Here's how the part is built. I have some questions about the finished solid (model axes, mm). A direction names the side the tool comes from. Coordinates: 2 decimals unless noted, no trailing zeros. Loops run counter-clockwise (first coordinate to the right, second up) from the corner with the lowest first, then second, coordinate; pieces in that order, holes last. Notation, with made-up numbers: (54, 18) - (68, 18) arc R33 ccw to (68, 56) - close; hole circle Ø3 at (48.25, 87.5). An arc over 180 degrees is marked (long way). Use a Markdown table: item, result.
```python
from build123d import *

# Parameters (mm, degrees)
BOX_W                     = 0.6
BOX_H                     = 0.4
BOX_DEPTH                 = 2.5
BOX001_W                  = 0.6
BOX001_H                  = 0.4
BOX001_DEPTH              = 2.5
CYLINDER011_R             = 5.5
CYLINDER011_DEPTH         = 2
BOX002_W                  = 6
BOX002_H                  = 15
BOX002_DEPTH              = 0.5
FILLET006_R               = 0.3
FUSION004_PLACEMENT_ANGLE = 90


with BuildPart() as cubo001:
    # Box → Box (new body)
    with BuildSketch(Plane(origin=(2.95, -0.2, -2), x_dir=(1, 0, 0), z_dir=(0, 0, 1))):
        with Locations((0.3, 0.2)):
            Rectangle(BOX_W, BOX_H)
    extrude(amount=BOX_DEPTH)


with BuildPart() as cubo002:
    # Box001 → Box001 (new body)
    with BuildSketch(Plane(origin=(-3.55, -0.2, -2), x_dir=(1, 0, 0), z_dir=(0, 0, 1))):
        with Locations((0.3, 0.2)):
            Rectangle(BOX001_W, BOX001_H)
    extrude(amount=BOX001_DEPTH)


with BuildPart() as interior:
    # Cylinder011 → Cylinder011 (new body)
    with BuildSketch(Plane.XY):
        Circle(CYLINDER011_R)
    extrude(amount=CYLINDER011_DEPTH)

    # Fusion: union Cubo001, Cubo002
    add(cubo001.part)
    add(cubo002.part)


with BuildPart() as interior_1:
    # Fusion placement: moved
    add(interior.part.moved(Location((0, 0, 0.5))))


with BuildPart() as cubo:
    # Box002 → Box002 (new body)
    with BuildSketch(Plane(origin=(-3, -7, 0), x_dir=(1, 0, 0), z_dir=(0, 0, 1))):
        with Locations((3, 7.5)):
            Rectangle(BOX002_W, BOX002_H)
    extrude(amount=BOX002_DEPTH)


with BuildPart() as obj1:
    # Sketch004 → Revolution001 (revolve)
    with BuildSketch(Plane.XZ):
        Polygon((5.5, 2.5), (5.5, 0), (6, 0), (6, 2), (5.75, 2), (5.75, 2.5), align=None)
    revolve(axis=Axis((0, 0, 0), (0, 0, 1)))

    # Cut013: cut Cubo
    add(cubo.part, mode=Mode.SUBTRACT)


with BuildPart() as buzzersensor:
    # Sketch003 → Revolution (revolve)
    with BuildSketch(Plane.XZ):
        Polygon((1.3, 9.57124), (6, 9.57124), (6, 2.17124), (5.75, 2.17124), (5.75, 2.57124), (5.5, 2.57124), (5.5, 9.07124), (1.3, 9.07124), align=None)
    revolve(axis=Axis((0, 0, 0), (0, 0, 1)))

    # Fillet006
    fillet006_edges = [buzzersensor.edges().sort_by_distance(p)[0] for p in [
        (-6, 0, 9.57124),
    ]]
    fillet(fillet006_edges, radius=FILLET006_R)

    # Fusion004: union Interior, obj1
    add(interior_1.part)
    add(obj1.part)


with BuildPart() as buzzersensor_1:
    # Fusion004 placement: moved
    add(buzzersensor.part.moved(Location((6, 2.7, 1))).rotate(Axis((6, 2.7, 1), (0, 0, 1)), FUSION004_PLACEMENT_ANGLE))


solid = buzzersensor_1.part
```
Q1. Please list where these lines run through material, in increasing order: L1, parallel to Z at x = 3.25, y = 5.75; L2, parallel to X at y = 2.7, z = 10.25; L3, parallel to X at y = 2.7, z = 8.5. Write a range as from..to.
Check values:
| item | result |
|---|---|
| L1 | 1.5..3.5, 10.07..10.57 |
| L2 | 0..4.7, 7.3..12 |
| L3 | 0..0.5, 11.5..12 |
Q2. Which directions (+Z, -Z, +X, -X, +Y, -Y) give clear straight access to the entire face, cutting with the end or side of a thin tool? Please do faces 1 (the face through (6, 1, 10.071)), 2 (the face through (6.1, 8.2, 1.2)), 3 (the face through (7.27, 2.42, 10.32)), 4 (the face through (11.323, 5.469, 6.672)).
Check values:
| item | result |
|---|---|
| face 1 | none |
| face 2 | -Z |
| face 3 | +Z |
| face 4 | +Z, -Z |
Q3. Will these pins go through, and if not, where does the flat tip stop? P1, Ø0.6, axis at x = 11, z = 1.5, coming from the -Y side; P2, Ø0.5, axis at y = 6, z = 0, coming from the -X side; P3, Ø3, axis at x = 8, z = 8.5, coming from the +Y side.
Check values:
| item | result |
|---|---|
| P1 | y = -1.03 |
| P2 | x = 5.8 |
| P3 | y = 8.68 |
Q4. I want a section at A-A, the plane y = 2.7. Write out the boundary of the cut face in (x, z), then the cut area to 3 significant figures.
Check values:
| item | result |
|---|---|
| outline | (0, 1.5) - (12, 1.5) - (12, 3) - (11.75, 3) - (11.75, 3.17) - (12, 3.17) - (12, 10.27) arc R0.3 ccw to (11.7, 10.57) - (7.3, 10.57) - (7.3, 10.07) - (11.5, 10.07) - (11.5, 3.57) - (11.75, 3.57) - (11.75, 3.5) - (0.25, 3.5) - (0.25, 3.57) - (0.5, 3.57) - (0.5, 10.07) - (4.7, 10.07) - (4.7, 10.57) - (0.3, 10.57) arc R0.3 ccw to (0, 10.27) - (0, 3.17) - (0.25, 3.17) - (0.25, 3) - (0, 3) - close |
| area | 35.1 mm^2 |
Q5. If we mould it in two halves opening along X, with no side actions, what happens to faces 5 (the face through (6, 3, 1.5)), 6 (the face through (7.2, 1.5, 10.571)), 7 (the face through (0.05, 1.92, 2.01))? For each: pulls with the +X half, pulls with the -X half, needs draft (parallel to the pull), parting line crosses it, or undercut.
Check values:
| item | result |
|---|---|
| face 5 | undercut |
| face 6 | needs draft |
| face 7 | parting line crosses it |
Q6. I want a section at B-B, the plane z = 8. Write out the boundary of the cut face in (x, y).
Check values:
| item | result |
|---|---|
| outline | circle Ø12 at (6, 2.7); hole circle Ø11 at (6, 2.7) |
